Verification items for the finished model (mm, model axes). Give positions to 0.01 mm unless a question says otherwise; leave off trailing zeros. Write each loop counter-clockwise with the first axis right and the second up, starting at its lowest first coordinate (ties: lowest second). Pieces come first, ordered by that corner, then holes. Notation, with made-up numbers: (63, 17) -> (107, 17) arc R12 cw to (107, 28) -> close; hole circle Ø2 at (4.25, 31). An arc over 180 degrees is marked (long way). Write item = value, one per line.
Autodesk Inventor part; units mm, degrees
ref_plane "YZ Plane" through (0, 0, 0) normal (1, 0, 0) x (0, 1, 0)
ref_plane "XZ Plane" through (0, 0, 0) normal (0, 1, 0) x (-1, 0, 0)
ref_plane "XY Plane" through (0, 0, 0) normal (0, 0, 1) x (1, 0, 0)
sketch "Эскиз4" plane through (0, 0, 0) normal (0, 0, 1) x (1, 0, 0)
  line L0 (1, -3.5) -> (-1, -3.5)
  line L1 (-2.5, -2) -> (-2.5, 2)
  line L2 (-1, 3.5) -> (1, 3.5)
  line L3 (2.5, 2) -> (2.5, -2)
  line L4 (2.5, -3.5) -> (-2.5, 3.5) construction
  line L5 (-2.5, -3.5) -> (2.5, 3.5) construction
  arc A0 (2.5, 2) -> (1, 3.5) centre (1, 2) ccw
  arc A1 (-1, 3.5) -> (-2.5, 2) centre (-1, 2) ccw
  arc A2 (-2.5, -2) -> (-1, -3.5) centre (-1, -2) ccw
  arc A3 (1, -3.5) -> (2.5, -2) centre (1, -2) ccw
  point P0 (0, 0)
  point P1 (0, -3)
  point P2 (0, 3)
  dimension "d15" = 5
  dimension "d16" = 7
  dimension "d17" = 1.5
  dimension "d18" = 1.5
extrude "Выдавливание2" add sketch "Эскиз4" along normal blind 10
properties part number "Clemm"
Item 1: Go/stop test with a flat-tipped pin: P1, Ø1.5, axis at x = 0, y = 1, coming from the -Z side. Record where the tip stops, or that it passes through.
Response values:
P1 = 0
Item 2: Sectioned sample at A-A on z = 2.25. Record the cut outline in (x, y).
Response values:
outline = (-2.5, -2) arc R1.5 ccw to (-1, -3.5) -> (1, -3.5) arc R1.5 ccw to (2.5, -2) -> (2.5, 2) arc R1.5 ccw to (1, 3.5) -> (-1, 3.5) arc R1.5 ccw to (-2.5, 2) -> close
Item 3: Material ranges on line 1 (Y direction, x = 1.1, z = 7.75); line 2 (X direction, y = -3, z = 7.5); line 3 (Y direction, x = -1.6, z = 5), recorded low to high.
Response values:
line_1 = -3.5 to 3.5
line_2 = -2.12 to 2.12
line_3 = -3.37 to 3.37
Item 4: Sectioned sample at B-B on x = 2.25. Record the cut outline in (y, z), then the cut area to 3 significant figures.
Response values:
outline = (-2.83, 0) -> (2.83, 0) -> (2.83, 10) -> (-2.83, 10) -> close
area = 56.6 mm^2
Item 5: Sectioned sample at C-C on y = -2.5. Record the cut outline in (x, z).
Response values:
outline = (-2.41, 0) -> (2.41, 0) -> (2.41, 10) -> (-2.41, 10) -> close
